from build123d import *

# Parameters (mm, degrees)
BOSS_EXTRUDE1_DEPTH   = 4.7625
CUT_EXTRUDE1_DEPTH    = 5.7625
CUT_EXTRUDE2_DEPTH    = 5.7625
FILLET1_R             = 1
SKETCH4_R             = 4
BOSS_EXTRUDE3_DEPTH   = 4.7625
SKETCH5_R             = 3.125
CUT_EXTRUDE3_DEPTH    = 5.7625
SKETCH6_R             = 3.5
CUT_EXTRUDE4_DEPTH    = 3.2625
SKETCH7_R             = 6.5
CUT_EXTRUDE5_DEPTH    = 5.7625
SKETCH8_R             = 7
CUT_EXTRUDE6_DEPTH    = 3.2625
M3X0_5_TAPPED_HOLE1_D = 2.5
M3X0_5_TAPPED_HOLE2_D = 2.5


with BuildPart() as part:
    # Sketch1 → Boss-Extrude1 (new body)
    with BuildSketch(Plane(origin=(0, 0, 0), x_dir=(1, 0, 0), z_dir=(0, 1, 0))):
        with BuildLine():
            Line((-35, 14.5), (19.483879351, 14.5))
            ThreePointArc((19.483879351, 14.5), (22.269309423, 14.89576243), (24.834265782, 16.051724138))
            ThreePointArc((24.834265782, 16.051724138), (54, 0), (24.834265782, -16.051724138))
            ThreePointArc((24.834265782, -16.051724138), (22.269309423, -14.89576243), (19.483879351, -14.5))
            Line((19.483879351, -14.5), (-35, -14.5))
            ThreePointArc((-35, -14.5), (-49.5, 0), (-35, 14.5))
        make_face()
    extrude(amount=BOSS_EXTRUDE1_DEPTH)

    # Sketch2 → Cut-Extrude1 (cut, through all)
    with BuildSketch(Plane(origin=(0, 4.7625, 0), x_dir=(1, 0, 0), z_dir=(0, 1, 0))):
        with BuildLine():
            Line((-35, 14.5), (27.609823933, 17.503865221))
            ThreePointArc((27.609823933, 17.503865221), (25.539879113, 16.477442544), (23.609823933, 15.207362991))
            ThreePointArc((23.609823933, 15.207362991), (-1.577083946, 6.065910022), (-27.59576752, 12.467050228))
            ThreePointArc((-27.59576752, 12.467050228), (-31.160874338, 13.98252889), (-35, 14.5))
        make_face()
    extrude(amount=-CUT_EXTRUDE1_DEPTH, mode=Mode.SUBTRACT)

    # Sketch3 → Cut-Extrude2 (cut, through all)
    with BuildSketch(Plane(origin=(0, 4.7625, 0), x_dir=(1, 0, 0), z_dir=(0, 1, 0))):
        with BuildLine():
            Line((-25, -10.5), (-8.18305643, -10.5))
            Line((-8.18305643, -10.5), (-21.431362429, 5.11293208))
            ThreePointArc((-21.431362429, 5.11293208), (-20.86454524, -3.230931556), (-25, -10.5))
        make_face()
        with BuildLine():
            Line((-14.47546762, 3.097845852), (-2.937056907, -10.5))
            Line((-2.937056907, -10.5), (9.456330798, 3.851674059))
            ThreePointArc((9.456330798, 3.851674059), (-2.463897631, 2.02484882), (-14.47546762, 3.097845852))
        make_face()
        with BuildLine():
            Line((17.235698957, 6.740148995), (2.347968808, -10.5))
            Line((2.347968808, -10.5), (19.164912378, -10.5))
            ThreePointArc((19.164912378, -10.5), (16.117854624, -2.112956696), (17.235698957, 6.740148995))
        make_face()
    extrude(amount=-CUT_EXTRUDE2_DEPTH, mode=Mode.SUBTRACT)

    # Fillet1
    fillet1_edges = [part.edges().sort_by_distance(p)[0] for p in [
        (17.235698957, 2.38125, -6.740148995),
        (19.164912378, 2.38125, 10.5),
        (2.347968808, 2.38125, 10.5),
        (-21.431362429, 2.38125, -5.11293208),
        (-8.18305643, 2.38125, 10.5),
        (-25, 2.38125, 10.5),
        (-14.47546762, 2.38125, -3.097845852),
        (9.456330798, 2.38125, -3.851674059),
        (-2.937056907, 2.38125, 10.5),
    ]]
    fillet(fillet1_edges, radius=FILLET1_R)

    # Sketch4 → Boss-Extrude3 (add, through all)
    with BuildSketch(Plane(origin=(0, 4.7625, 0), x_dir=(1, 0, 0), z_dir=(0, 1, 0))):
        with Locations((-35, 0)):
            Circle(SKETCH4_R)
    extrude(amount=-BOSS_EXTRUDE3_DEPTH)

    # Sketch5 → Cut-Extrude3 (cut, through all)
    with BuildSketch(Plane(origin=(0, 4.7625, 0), x_dir=(1, 0, 0), z_dir=(0, 1, 0))):
        with Locations((-35, 0)):
            Circle(SKETCH5_R)
    extrude(amount=-CUT_EXTRUDE3_DEPTH, mode=Mode.SUBTRACT)

    # Sketch6 → Cut-Extrude4 (cut)
    with BuildSketch(Plane(origin=(0, 0, 0), x_dir=(1, 0, 0), z_dir=(0, 1, 0))):
        with Locations((-35, 0)):
            Circle(SKETCH6_R)
    extrude(amount=CUT_EXTRUDE4_DEPTH, mode=Mode.SUBTRACT)

    # Sketch7 → Cut-Extrude5 (cut, through all)
    with BuildSketch(Plane.XZ):
        with Locations((35, 0)):
            Circle(SKETCH7_R)
    extrude(amount=-CUT_EXTRUDE5_DEPTH, mode=Mode.SUBTRACT)

    # Sketch8 → Cut-Extrude6 (cut)
    with BuildSketch(Plane.XZ):
        with Locations((35, 0)):
            Circle(SKETCH8_R)
    extrude(amount=-CUT_EXTRUDE6_DEPTH, mode=Mode.SUBTRACT)

    # M3x0.5 Tapped Hole1 (through all)
    with Locations(Plane.XZ):
        with Locations((27.75, -12.557368355), (27.75, 12.557368355), (49.5, 0), (-44, 0), (-30.5, 7.794228634), (-30.5, -7.794228634)):
            Hole(M3X0_5_TAPPED_HOLE1_D / 2)

    # M3x0.5 Tapped Hole2 (through all)
    with Locations(Plane(origin=(0, 4.7625, 0), x_dir=(-1, 0, 0), z_dir=(0, 1, 0))):
        with Locations((30.5, 7.794228634), (44, 0), (30.5, -7.794228634)):
            Hole(M3X0_5_TAPPED_HOLE2_D / 2)


solid = part.part
Can you work these out from the model? Positions are in its coordinate system, mm. A direction names the side the tool comes from. Round coordinates to 2 decimals unless told otherwise and drop trailing zeros. Loops run counter-clockwise (first coordinate to the right, second up) from the corner with the lowest first, then second, coordinate; pieces in that order, holes last. Notation, with made-up numbers: (-7.75, -23.75) - (49.25, -23.75) arc R24 ccw to (49.25, 2.25) - close; hole circle Ø3 at (52.5, -38). An arc over 180 degrees is marked (long way). Answer in a Markdown table with one row per item. Add a question column.
Q1. For pin 1 Ø1.4 at (x, y) = (10, 2) entering from -Z; pin 2 Ø2 at (x, y) = (19, 1) entering from -Z; pin 3 Ø1 at (y, z) = (4, 9.5) entering from -X, each with a flat end and sliding along its axis, tell me the tip position at first contact or that it passes through.
Q2. I want a section at C-C on y = 1.25. Count the separate pieces of the cut face and the enclosed holes in it, and give its area (3 significant figures).
Q3. Which directions (+Z, -Z, +X, -X, +Y, -Y) give clear straight access to the entire face, cutting with the end or side of a thin tool? Please do faces 5 (the cylindrical face through (-38.497, 1.608, -0.154)), 6 (the cylindrical face through (-19.96, 2.35, -2.28)).
Q4. I want a section at B-B on x = -30.5. List the corners of the cut face in (y, z) for me.
Q5. I want a section at A-A on x = 31.5. List the corners of the cut face in (y, z) for me.
Q6. I want a section at D-D on x = -16. List the corners of the cut face in (y, z) for me.
Q7. We'd pull the mould along Z, two halves only. Please class faces 1 (the cylindrical face through (50.49, 2.41, -0.76)), 2 (the flat face through (-7, 2, 14.5)), 3 (the flat face through (3, 4.762, 4)), 4 (the cylindrical face through (-31.655, 2.415, -8.273)): pulls with the +Z half, pulls with the -Z half, needs draft (parallel to the pull), parting line crosses it, or undercut.
Q8. I need wall thicknesses on L1, parallel to Z at x = 35, y = 4.1; L2, parallel to X at y = 1.55, z = 8.5; L3, parallel to Z at x = 27.75, y = 2.95. Which ranges of each line are inside material? Lowest first, please.
A:
| question | item | result |
|---|---|---|
| 1 | pin 1 | z = -8.42 |
| 1 | pin 2 | z = -12.76 |
| 1 | pin 3 | x = -46.37 |
| 2 | separate pieces | 1 |
| 2 | enclosed holes | 11 |
| 2 | area | 2,120 mm^2 |
| 3 | face 5 | -Y |
| 3 | face 6 | +Y, -Y |
| 4 | outline | (0, -13.78) - (4.76, -13.78) - (4.76, -9.04) - (0, -9.04) - close; (0, -6.54) - (4.76, -6.54) - (4.76, 6.54) - (0, 6.54) - close; (0, 9.04) - (4.76, 9.04) - (4.76, 14.5) - (0, 14.5) - close |
| 5 | outline | (0, -18.67) - (4.76, -18.67) - (4.76, -5.48) - (3.26, -5.48) - (3.26, -6.06) - (0, -6.06) - close; (0, 6.06) - (3.26, 6.06) - (3.26, 5.48) - (4.76, 5.48) - (4.76, 18.67) - (0, 18.67) - close |
| 6 | outline | (0, -7.58) - (4.76, -7.58) - (4.76, 1.29) - (0, 1.29) - close; (0, 10.5) - (4.76, 10.5) - (4.76, 14.5) - (0, 14.5) - close |
| 7 | face 1 | undercut |
| 7 | face 2 | pulls with the +Z half |
| 7 | face 3 | needs draft |
| 7 | face 4 | undercut |
| 8 | L1 | -19 to -6.5, 6.5 to 19 |
| 8 | L2 | -46.75 to -31.53, -29.47 to -23.25, -9.88 to -4.63, -1.21 to 4.08, 18.01 to 51.99 |
| 8 | L3 | -17.56 to -13.81, -11.31 to 11.31, 13.81 to 17.56 |
